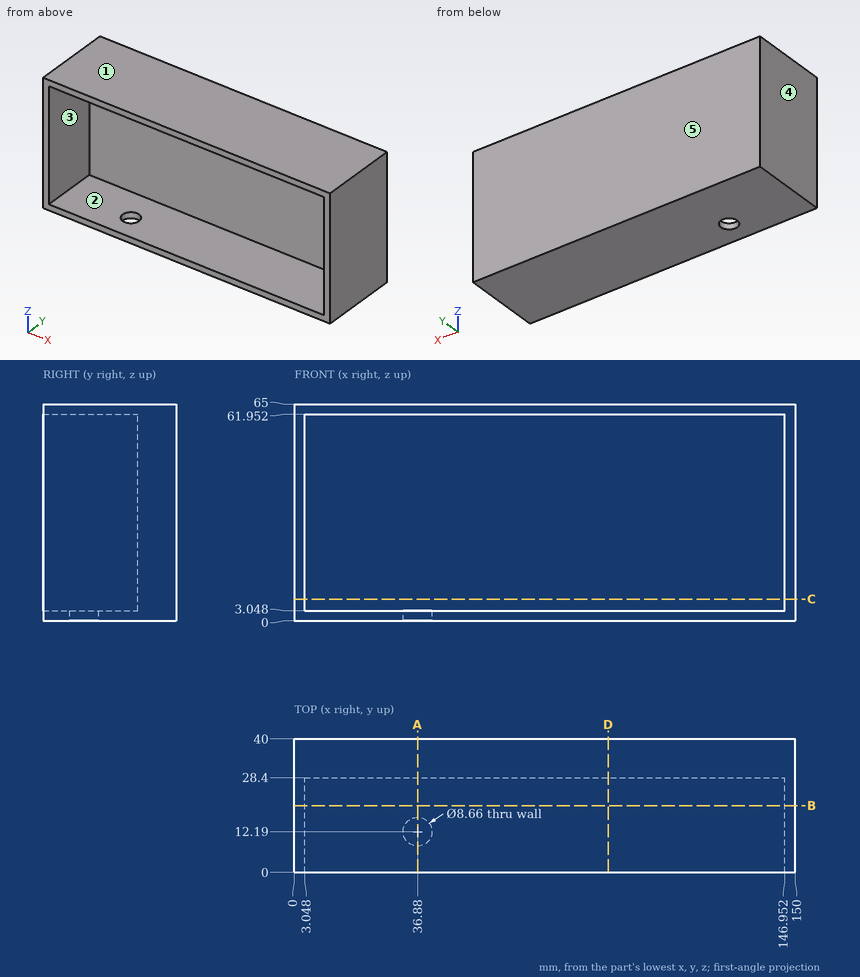
Geometry: see drawing. Coordinates: mm, zero at the bounding-box minimum. A direction names the side the tool comes from. Give positions to 0.01 mm unless a question says otherwise; leave off trailing zeros. Order: outer loops, then holes, each group sorted by start corner. A loop starts at its lowest first (then second) coordinate and runs counter-clockwise, first axis right, second up. Notation, with made-up numbers: (15.25, 82.25) -> (55.25, 82.25) arc R12 ccw to (55.25, 93.25) -> close; hole circle Ø6 at (21, 50.25). An arc over 180 degrees is marked (long way). Write each question's results on one line, items separated by ' | '.
1) Line query: line 1 along X through (y, z) = (12, 2); line 2 along Z through (x, y) = (82, 17.5); line 3 along X through (y, z) = (10, 36). Output: solid intervals per line, ascending.
Geometry says:
line 1: x = 0 to 32.55, 41.21 to 150 | line 2: z = 0 to 3.05, 61.95 to 65 | line 3: x = 0 to 3.05, 146.95 to 150
2) Cut plane C-C (z = 6.5). Output: boundary loops of the cut face in (x, y).
Geometry says:
outline: (0, 0) -> (3.05, 0) -> (3.05, 28.4) -> (146.95, 28.4) -> (146.95, 0) -> (150, 0) -> (150, 40) -> (0, 40) -> close
3) Set-up query: the marked faces 1 and 2. Return all of +Z, -Z, +X, -X, +Y, -Y with unobstructed straight access to the full face (end or side cutting, diameter ignored); none if empty.
Geometry says:
face 1: +Z, +X, -X, +Y, -Y | face 2: -Y
4) Cut plane D-D (x = 94). Output: boundary loops of the cut face in (y, z), and give its area (3 significant figures).
Geometry says:
outline: (0, 0) -> (40, 0) -> (40, 65) -> (0, 65) -> (0, 61.95) -> (28.4, 61.95) -> (28.4, 3.05) -> (0, 3.05) -> close | area: 927 mm²
5) Cut plane A-A (x = 36.88). Output: boundary loops of the cut face in (y, z), and give its area (3 significant figures).
Geometry says:
outline: (0, 0) -> (7.86, 0) -> (7.86, 3.05) -> (0, 3.05) -> close; (0, 61.95) -> (28.4, 61.95) -> (28.4, 3.05) -> (16.52, 3.05) -> (16.52, 0) -> (40, 0) -> (40, 65) -> (0, 65) -> close | area: 901 mm²
6) Cut plane B-B (y = 20). Output: boundary loops of the cut face in (x, z).
Geometry says:
outline: (0, 0) -> (150, 0) -> (150, 65) -> (0, 65) -> close; hole (3.05, 3.05) -> (146.95, 3.05) -> (146.95, 61.95) -> (3.05, 61.95) -> close
7) Draft query along X for the marked faces 3, 4 and 5. Return one class per face: released by +X, released by -X, zero draft, split by the parting line, or undercut.
Geometry says:
face 3: undercut | face 4: released by -X | face 5: zero draft
8) First-contact query: pin 1 Ø5 at (x, z) = (120, 45.5) entering from -Y; pin 2 Ø8 at (x, y) = (36.88, 12.19) entering from -Z. Flat tips, straight axial feed; report the tip coordinate or a pass-through.
Geometry says:
pin 1: stops at y = 28.4 | pin 2: stops at z = 61.95
